Design review of the part built by this model. Coordinates are the model's own, in mm. A direction names the side the tool comes from. Round coordinates to 2 decimals unless told otherwise and drop trailing zeros. Order: outer loops, then holes, each group sorted by start corner. A loop starts at its lowest first (then second) coordinate and runs counter-clockwise, first axis right, second up. Notation, with made-up numbers: (-26.75, -26) - (12.25, -26) arc R20 cw to (12.25, -4) - close; hole circle Ø3 at (71, -26.75). An arc over 180 degrees is marked (long way). Write item = value, one per line.
from build123d import *

# Parameters (mm, degrees)
SKETCH1_W                 = 76.2
SKETCH1_H                 = 63.5
SKETCH1_W_2               = 50.280812534
SKETCH1_H_2               = 38.222705752
BOSS_EXTRUDE1_DEPTH       = 1.5
FILLET1_R                 = 3.175
F_4_CLEARANCE_HOLE1_D     = 3.2639
F_4_CLEARANCE_HOLE1_DEPTH = 6.619425513
F_4_CLEARANCE_HOLE1_TIP   = 0.980574487


with BuildPart() as part:
    # Sketch1 → Boss-Extrude1 (new body, symmetric)
    with BuildSketch(Plane(origin=(0, 0, 0), x_dir=(1, 0, 0), z_dir=(0, 1, 0))):
        Rectangle(SKETCH1_W, SKETCH1_H)
        Rectangle(SKETCH1_W_2, SKETCH1_H_2, mode=Mode.SUBTRACT)
    extrude(amount=BOSS_EXTRUDE1_DEPTH, both=True)

    # Fillet1
    fillet1_edges = [part.edges().sort_by_distance(p)[0] for p in [
        (25.140406267, 0, 19.111352876),
        (25.140406267, 0, -19.111352876),
        (-25.140406267, 0, -19.111352876),
        (-25.140406267, 0, 19.111352876),
        (38.1, 0, 31.75),
        (-38.1, 0, 31.75),
        (-38.1, 0, -31.75),
        (38.1, 0, -31.75),
    ]]
    fillet(fillet1_edges, radius=FILLET1_R)

    # #4 Clearance Hole1
    with Locations(Plane(origin=(0, 1.5, 0), x_dir=(1, 0, 0), z_dir=(0, 1, 0))):
        with Locations((-34.125, 0), (-30.315, -23.045), (0, -26.77), (30.315, -23.045), (34.125, 0), (30.315, 23.045), (0, 26.77), (-30.315, 23.045)):
            Hole(F_4_CLEARANCE_HOLE1_D / 2, depth=F_4_CLEARANCE_HOLE1_DEPTH)
            with Locations((0, 0, -(F_4_CLEARANCE_HOLE1_DEPTH + F_4_CLEARANCE_HOLE1_TIP / 2))):  # 118° drill point
                Cone(0, F_4_CLEARANCE_HOLE1_D / 2, F_4_CLEARANCE_HOLE1_TIP, mode=Mode.SUBTRACT)


solid = part.part
Item 1: For faces 1 (the face through (0, 0, 31.75)), 2 (the face through (0, 0, -19.111)), list the 3-axis set-ups (+Z, -Z, +X, -X, +Y, -Y) from which the entire face can be reached by the end or side of a thin tool; tool diameter is ignored.
Data:
face_1 = +Z, +X, -X, +Y, -Y
face_2 = +Y, -Y
Item 2: Take a section at A-A, the plane z = 13. State the section outline as (x, y) points, and give its area (3 significant figures).
Data:
outline = (-38.1, -1.5) - (-25.14, -1.5) - (-25.14, 1.5) - (-38.1, 1.5) - close; (25.14, -1.5) - (38.1, -1.5) - (38.1, 1.5) - (25.14, 1.5) - close
area = 77.8 mm2
Item 3: For line 1 along Z through (x, y) = (17, 0.75); line 2 along X through (y, z) = (0.45, 2.5); line 3 along Z through (x, y) = (0, -0.1), list the stretches that pass through material, from the lowest coordinate up. Write a range as [from, to].
Data:
line_1 = [-31.75, -19.11], [19.11, 31.75]
line_2 = [-38.1, -25.14], [25.14, 38.1]
line_3 = [-31.75, -28.4], [-25.14, -19.11], [19.11, 25.14], [28.4, 31.75]
Item 4: Take a section at C-C, the plane z = 0. State the section outline as (x, y) points, and give its area (3 significant figures).
Data:
outline = (-38.1, -1.5) - (-35.76, -1.5) - (-35.76, 1.5) - (-38.1, 1.5) - close; (-32.49, -1.5) - (-25.14, -1.5) - (-25.14, 1.5) - (-32.49, 1.5) - close; (25.14, -1.5) - (32.49, -1.5) - (32.49, 1.5) - (25.14, 1.5) - close; (35.76, -1.5) - (38.1, -1.5) - (38.1, 1.5) - (35.76, 1.5) - close
area = 58.2 mm2
Item 5: The part is to be moulded in two halves that separate along Z. For faces 3 (the face through (-1, -1.5, -22)), 4 (the face through (24.235, -0.021, 18.157)), 5 (the face through (-37.19, -0.02, -30.8)), say which applies: +Z half, -Z half, draft (parallel to the pull), parting line (faces both ways), or undercut.
Data:
face_3 = draft
face_4 = undercut
face_5 = -Z half
Item 6: Take a section at B-B, the plane x = 12.5. State the section outline as (y, z) points, and give its area (3 significant figures).
Data:
outline = (-1.5, -31.75) - (1.5, -31.75) - (1.5, -19.11) - (-1.5, -19.11) - close; (-1.5, 19.11) - (1.5, 19.11) - (1.5, 31.75) - (-1.5, 31.75) - close
area = 75.8 mm2
Item 7: Take a section at D-D, the plane x = 0. State the section outline as (y, z) points, and give its area (3 significant figures).
Data:
outline = (-1.5, -31.75) - (1.5, -31.75) - (1.5, -28.4) - (-1.5, -28.4) - close; (-1.5, -25.14) - (1.5, -25.14) - (1.5, -19.11) - (-1.5, -19.11) - close; (-1.5, 19.11) - (1.5, 19.11) - (1.5, 25.14) - (-1.5, 25.14) - close; (-1.5, 28.4) - (1.5, 28.4) - (1.5, 31.75) - (-1.5, 31.75) - close
area = 56.2 mm2
